Work out the finished part from the listing and answer in its coordinate system (mm). A direction names the side the tool comes from. Round coordinates to 2 decimals unless told otherwise and drop trailing zeros. Order: outer loops, then holes, each group sorted by start corner. A loop starts at its lowest first (then second) coordinate and runs counter-clockwise, first axis right, second up. Notation, with made-up numbers: M -6,34 L 40,34 A9 ccw 40,50 Z; hole C -11,71.25 d4. An arc over 180 degrees is marked long. Return JSON: item names as keys, results as strings.
from build123d import *

# Parameters (mm, degrees)
SKETCH1_R                   = 5.985
BOSS_EXTRUDE1_DEPTH         = 16
SKETCH2_R                   = 3.5
BOSS_EXTRUDE2_DEPTH         = 65
SKETCH3_W                   = 6
SKETCH3_H                   = 6
BOSS_EXTRUDE3_DEPTH         = 9
SKETCH4_R                   = 1.99
BOSS_EXTRUDE4_DEPTH         = 7
BOSS_EXTRUDE5_START         = 12
SKETCH5_R                   = 3.5
BOSS_EXTRUDE5_DEPTH         = 12
TAP_DRILL_FOR_M4_TAP1_D     = 3.3
TAP_DRILL_FOR_M4_TAP1_DEPTH = 9
TAP_DRILL_FOR_M4_TAP1_TIP   = 0.991420021
DOME1_FACE_RADIUS           = 1.99
DOME1_HEIGHT                = 1


with BuildPart() as part:
    # Sketch1 → Boss-Extrude1 (new body)
    with BuildSketch(Plane(origin=(0, 0, 0), x_dir=(1, 0, 0), z_dir=(0, 1, 0))):
        with Locations(Location((0, 0, 0), (0, 0, 270))):
            Circle(SKETCH1_R)
    extrude(amount=BOSS_EXTRUDE1_DEPTH)

    # Sketch2 → Boss-Extrude2 (add)
    with BuildSketch(Plane(origin=(0, 16, 0), x_dir=(1, 0, 0), z_dir=(0, 1, 0))):
        with Locations(Location((0, 0, 0), (0, 0, 270))):
            Circle(SKETCH2_R)
    extrude(amount=BOSS_EXTRUDE2_DEPTH)

    # Sketch3 → Boss-Extrude3 (add)
    with BuildSketch(Plane(origin=(0, 81, 0), x_dir=(1, 0, 0), z_dir=(0, 1, 0))):
        Rectangle(SKETCH3_W, SKETCH3_H)
    extrude(amount=BOSS_EXTRUDE3_DEPTH)

    # Sketch4 → Boss-Extrude4 (add)
    with BuildSketch(Plane(origin=(0, 90, 0), x_dir=(1, 0, 0), z_dir=(0, 1, 0))):
        with Locations(Location((0, 0, 0), (0, 0, 270))):
            Circle(SKETCH4_R)
    extrude(amount=BOSS_EXTRUDE4_DEPTH)

    # Sketch5 → Boss-Extrude5 (add)
    with BuildSketch(Plane.XZ.offset(BOSS_EXTRUDE5_START)):
        with Locations(Location((0, 0, 0), (0, 0, 238.997280866))):
            Circle(SKETCH5_R)
    extrude(amount=-BOSS_EXTRUDE5_DEPTH)

    # Tap Drill for M4 Tap1
    with Locations(Plane(origin=(0, -12, 0), x_dir=(-1, 0, 0), z_dir=(0, -1, 0))):
        with Locations((0, 0)):
            Hole(TAP_DRILL_FOR_M4_TAP1_D / 2, depth=TAP_DRILL_FOR_M4_TAP1_DEPTH)
            with Locations((0, 0, -(TAP_DRILL_FOR_M4_TAP1_DEPTH + TAP_DRILL_FOR_M4_TAP1_TIP / 2))):  # 118° drill point
                Cone(0, TAP_DRILL_FOR_M4_TAP1_D / 2, TAP_DRILL_FOR_M4_TAP1_TIP, mode=Mode.SUBTRACT)

    # Dome1: a dome of height H over a round flat face of radius A is a cap of a sphere of radius (A * A + H * H) / (2 * H)
    dome1_r = (DOME1_FACE_RADIUS * DOME1_FACE_RADIUS + DOME1_HEIGHT * DOME1_HEIGHT) / (2 * DOME1_HEIGHT)
    dome1_base = Plane((0, 97, 0), z_dir=(0, 1, 0))
    with Locations(dome1_base.offset(DOME1_HEIGHT - dome1_r)):
        dome1_ball = Sphere(dome1_r, mode=Mode.PRIVATE)
    add(split(dome1_ball, bisect_by=dome1_base, keep=Keep.TOP, mode=Mode.PRIVATE))


solid = part.part
Item 1: The mould has two halves that part along X. Classify faces 1 (the flat face through (3, 85, 0)), 2 (the cylindrical face through (-1.216, -7.437, -1.115)), 3 (the flat face through (-2, -12, 0)), 4 (the cylindrical face through (1.973, 93.451, -0.259)): pulls with the +X half, pulls with the -X half, needs draft (parallel to the pull), parting line crosses it, or undercut.
Output:
{"face 1": "pulls with the +X half", "face 2": "undercut", "face 3": "needs draft", "face 4": "parting line crosses it"}
Item 2: Consider line 1 along Z through (x, y) = (0, -7.5); line 2 along Y through (x, z) = (0.75, -3.5); line 3 along Y through (x, z) = (-1.25, 2.75). Determine where each line is inside the solid, lowest interval first. Write a range as [from, to].
Output:
{"line 1": "z = [-3.5, -1.65], [1.65, 3.5]", "line 2": "y = [0, 16]", "line 3": "y = [-12, 90]"}
Item 3: Find section A-A (y = -4). Determine the outline of the cut face in (x, z), plus the area to 3 significant figures.
Output:
{"outline": "C 0,0 d7; hole C 0,0 d3.3", "area": "29.9 mm^2"}
Item 4: Find section C-C (x = 4.75). Determine the outline of the cut face in (y, z).
Output:
{"outline": "M 0,-3.64 L 16,-3.64 L 16,3.64 L 0,3.64 Z"}
Item 5: Each of these flat-tipped pins is pushed along its axis until it touches: pin 1 (4 mm diameter, centred on x = 1.5, y = 50.5, fed in from -Z); pin 2 (0.6 mm diameter, centred on x = -1, z = 3, fed in from +Y); pin 3 (0.6 mm diameter, centred on x = 0, z = -3.5, fed in from +Y). Where does it stop, or does it pass through?
Output:
{"pin 1": "stops at z = -3.5", "pin 2": "stops at y = 90", "pin 3": "stops at y = 81"}
Item 6: Which of the six approach directions +Z, -Z, +X, -X, +Y, -Y give full straight-line access (tool end or side, diameter ignored) to faces 5 (the flat face through (0, 85, -3)), 6 (the flat face through (0, 85, 3)), 7 (the flat face through (-3, 85, 0))?
Output:
{"face 5": "-Z, +X, -X, +Y", "face 6": "+Z, +X, -X, +Y", "face 7": "+Z, -Z, -X, +Y"}
Item 7: Find section B-B (y = 27). Determine the outline of the cut face in (x, z), plus the area to 3 significant figures.
Output:
{"outline": "C 0,0 d7", "area": "38.5 mm^2"}
